from build123d import *

# Parameters (mm, degrees)
BOSS_EXTRUDE1_DEPTH     = 18
CUT_EXTRUDE1_DEPTH      = 18
EXTRUDE_THIN1_DEPTH     = 25
CUT_EXTRUDE2_DEPTH      = 77.021378572
CUT_EXTRUDE2_DEPTH_BACK = 77.021378572
SKETCH3_R               = 2.5
CHAMFER1_SIZE           = 1
CUT_EXTRUDE3_DEPTH      = 65.02538559
CUT_EXTRUDE3_DEPTH_BACK = 65.02538559
SKETCH6_R               = 2.5
CHAMFER3_SIZE           = 1


with BuildPart() as part:
    # Sketch1 → Boss-Extrude1 (new body)
    with BuildSketch(Plane(origin=(0, 0, 0), x_dir=(1, 0, 0), z_dir=(0, 1, 0))):
        with BuildLine():
            Line((37.5, -10), (37.5, 10))
            Line((37.5, 10), (27.5, 20))
            Line((27.5, 20), (-17.5, 20))
            ThreePointArc((-17.5, 20), (-31.64213568, 14.142135567), (-37.5, -1.6e-07))
            ThreePointArc((-37.5, -1.6e-07), (-31.642135567, -14.14213568), (-17.5, -20))
            Line((-17.5, -20), (27.5, -20))
            Line((27.5, -20), (37.5, -10))
        make_face()
    extrude(amount=BOSS_EXTRUDE1_DEPTH)

    # Sketch2 → Cut-Extrude1 (cut)
    with BuildSketch(Plane.XZ):
        Polygon((24.5, 5), (24.5, -5), (20.964466094, -8.535533906), (10.964466094, -8.535533906), (7.428932188, -5), (7.428932188, 5), (10.964466094, 8.535533906), (20.964466094, 8.535533906), align=None)
    extrude(amount=-CUT_EXTRUDE1_DEPTH, mode=Mode.SUBTRACT)

    # Sketch4 → Extrude-Thin1 (add)
    with BuildSketch(Plane.XZ):
        with BuildLine():
            Line((-17.5, -32), (32.470562748, -32))
            Line((32.470562748, -32), (49.5, -14.970562748))
            Line((49.5, -14.970562748), (49.5, 14.970562748))
            Line((49.5, 14.970562748), (32.470562748, 32))
            Line((32.470562748, 32), (-17.5, 32))
            ThreePointArc((-17.5, 32), (-49.5, 0), (-17.5, -32))
        make_face()
        with BuildLine():
            Line((-17.5, -20), (27.5, -20))
            Line((27.5, -20), (37.5, -10))
            Line((37.5, -10), (37.5, 10))
            Line((37.5, 10), (27.5, 20))
            Line((27.5, 20), (-17.5, 20))
            ThreePointArc((-17.5, 20), (-37.5, 0), (-17.5, -20))
        make_face(mode=Mode.SUBTRACT)
    extrude(amount=-EXTRUDE_THIN1_DEPTH)

    # Sketch3 → Cut-Extrude2 (cut, two sides: drawn at the far end of the back side and taken through both)
    with BuildSketch(Plane.XY.offset(20).offset(-CUT_EXTRUDE2_DEPTH_BACK)):
        with Locations((15.964466094, 5.5)):
            Circle(SKETCH3_R)
    extrude(amount=CUT_EXTRUDE2_DEPTH + CUT_EXTRUDE2_DEPTH_BACK, mode=Mode.SUBTRACT)

    # Chamfer1
    chamfer1_edges = [part.edges().sort_by_distance(p)[0] for p in [
        (15.964466094, 0, 8.535533906),
        (9.196699141, 0, 6.767766953),
        (7.428932188, 0, 0),
        (9.196699141, 0, -6.767766953),
        (15.964466094, 0, -8.535533906),
        (22.732233047, 0, -6.767766953),
        (24.5, 0, 0),
        (22.732233047, 0, 6.767766953),
        (9.196699141, 18, 6.767766953),
        (7.428932188, 18, 0),
        (9.196699141, 18, -6.767766953),
        (15.964466094, 18, -8.535533906),
        (22.732233047, 18, -6.767766953),
        (24.5, 18, 0),
        (22.732233047, 18, 6.767766953),
        (15.964466094, 18, 8.535533906),
        (-49.5, 25, 0),
        (7.485281374, 25, 32),
        (40.985281374, 25, 23.485281374),
        (49.5, 25, 0),
        (40.985281374, 25, -23.485281374),
        (7.485281374, 25, -32),
        (13.464466094, 5.5, -32),
        (13.464466094, 5.5, 32),
    ]]
    chamfer(chamfer1_edges, length=CHAMFER1_SIZE)

    # Sketch6 → Cut-Extrude3 (cut, two sides: drawn at the far end of the back side and taken through both)
    with BuildSketch(Plane(origin=(0, 25, 0), x_dir=(1, 0, 0), z_dir=(0, 1, 0)).offset(-CUT_EXTRUDE3_DEPTH_BACK)):
        with Locations(Location((0, 25.5, 0), (0, 0, 270))):
            Circle(SKETCH6_R)
        with Locations(Location((0, -25.5, 0), (0, 0, 270))):
            Circle(SKETCH6_R)
        with Locations(Location((43, 0, 0), (0, 0, 270))):
            Circle(SKETCH6_R)
        with Locations(Location((-43, 0, 0), (0, 0, 270))):
            Circle(SKETCH6_R)
    extrude(amount=CUT_EXTRUDE3_DEPTH + CUT_EXTRUDE3_DEPTH_BACK, mode=Mode.SUBTRACT)

    # Chamfer3
    chamfer3_edges = [part.edges().sort_by_distance(p)[0] for p in [
        (0, 25, -28),
        (0, 25, 23),
        (43, 25, -2.5),
        (-43, 25, -2.5),
    ]]
    chamfer(chamfer3_edges, length=CHAMFER3_SIZE)


solid = part.part
Geometry check sheet. Reference: the model listing, model coordinates, mm. A direction names the side the tool comes from. Give positions to 0.01 mm unless a question says otherwise; leave off trailing zeros. Write each loop counter-clockwise with the first axis right and the second up, starting at its lowest first coordinate (ties: lowest second). Pieces come first, ordered by that corner, then holes. Notation, with made-up numbers: M 45.25,54 L 100.25,54 A20 ccw 100.25,73 Z; hole C 12,9 d11. An arc over 180 degrees is marked long. Answer as CSV lines item,"result". Start each with the question number.
Q1. Material ranges on L1, parallel to Z at x = 0, y = 12; L2, parallel to X at y = 5.5, z = -26.25; L3, parallel to X at y = 5.5, z = -24, recorded low to high.
Q2. Release check for a two-part mould opening along X. For faces 4 (the face through (-1, 0, 0)), 5 (the face through (23.06, 17.51, 7.16)), 6 (the face through (-49.492, 11.832, 0.704)) record: pulls with the +X half, pulls with the -X half, needs draft (parallel to the pull), parting line crosses it, or undercut.
Q3. Section check B-B, the plane z = 0. Give the number of separate pieces and of enclosed holes in the cut face, then the cut area to 3 significant figures.
Q4. Section check A-A, the plane y = 15. Record the cut outline in (x, z), then the cut area to 3 significant figures.
Q5. Tool access check on faces 1 (the face through (9.22, 8.89, -6.79)), 2 (the face through (5, 21, 20)), 3 (the face through (8.877, 0.507, -7.145)). Record the directions out of +Z, -Z, +X, -X, +Y, -Y that give a thin tool (end or side, any length) a straight path to the whole face; none if there is none.
Q6. Go/stop test with flat-tipped pins: pin 1 (2 mm diameter, centred on x = -20, z = 16, fed in from -Y); pin 2 (3 mm diameter, centred on y = 11.5, z = 2.5, fed in from -X); pin 3 (2 mm diameter, centred on y = 7.5, z = 11.5, fed in from -X); pin 4 (4 mm diameter, centred on y = 4, z = 22.5, fed in from -X). Record where each tip stops, or that it passes through.
Q7. Section check D-D, the plane x = 5. Record the cut outline in (y, z), then the cut area to 3 significant figures.
Geometry says:
1,L1,"-32 to -28, -23 to 23, 28 to 32"
1,L2,"-35.8 to -2.38, 2.38 to 13.46, 18.46 to 38.22"
1,L3,"-38.67 to -2, 2 to 13.46, 18.46 to 40.47"
2,face 4,"needs draft"
2,face 5,"undercut"
2,face 6,"pulls with the -X half"
3,separate pieces,"4"
3,enclosed holes,"0"
3,area,"1,390 mm^2"
4,outline,"M -17.5,-32 L 32.47,-32 L 49.5,-14.97 L 49.5,14.97 L 32.47,32 L -17.5,32 A32 ccw Z; hole C -43,0 d5; hole C 0,-25.5 d5; hole C 0,25.5 d5; hole M 7.43,-5 L 10.96,-8.54 L 20.96,-8.54 L 24.5,-5 L 24.5,5 L 20.96,8.54 L 10.96,8.54 L 7.43,5 Z; hole C 43,0 d5"
4,area,"5,260 mm^2"
5,face 1,"+Y, -Y"
5,face 2,"+Y"
5,face 3,"-Y"
6,pin 1,"y = 0"
6,pin 2,"x = -49.48"
6,pin 3,"x = -47.73"
6,pin 4,"x = -42.07"
7,outline,"M 0,-32 L 24,-32 L 25,-31 L 25,-20 L 18,-20 L 18,20 L 25,20 L 25,31 L 24,32 L 0,32 Z"
7,area,"1,320 mm^2"
